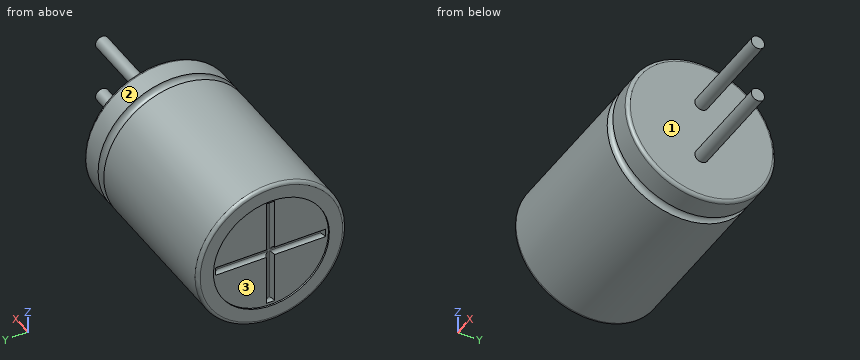
from build123d import *

# Parameters (mm, degrees)
SKETCH6_R           = 0.4
BOSS_EXTRUDE1_DEPTH = 6
CUT_EXTRUDE1_DEPTH  = 0.2
FILLET2_R           = 0.2


with BuildPart() as part:
    # Sketch1 → Revolve1 (revolve)
    with BuildSketch(Plane(origin=(0, 0, 0), x_dir=(1, 0, 0), z_dir=(0, 1, 0))):
        with BuildLine():
            Line((-5.95, -1.25), (-6.05, -1.25))
            Line((-6.05, -1.25), (-6.05, -2.25))
            Line((-6.05, -2.25), (-5.95, -2.25))
            Line((-5.95, -2.25), (3.85, -2.25))
            ThreePointArc((3.85, -2.25), (4.15, -1.95), (4.45, -2.25))
            Line((4.45, -2.25), (5.95, -2.25))
            Line((5.95, -2.25), (5.95, 2.25))
            Line((5.95, 2.25), (-5.95, 2.25))
            Line((-5.95, 2.25), (-5.95, -1.25))
        make_face()
    revolve(axis=Axis((-5.95, 0, -2.25), (1, 0, 0)))

    # Sketch6 → Boss-Extrude1 (add)
    with BuildSketch(Plane(origin=(5.95, 0, 0), x_dir=(0, 0, -1), z_dir=(1, 0, 0))):
        with Locations((0.5, 0)):
            Circle(SKETCH6_R)
        with Locations((4, 0)):
            Circle(SKETCH6_R)
    extrude(amount=BOSS_EXTRUDE1_DEPTH)

    # Sketch8 → Cut-Extrude1 (cut)
    with BuildSketch(Plane.ZY.offset(5.95)):
        Polygon((-2, -0.25), (-2, -3.325), (-2.5, -3.325), (-2.5, -0.25), (-5.575, -0.25), (-5.575, 0.25), (-2.5, 0.25), (-2.5, 3.325), (-2, 3.325), (-2, 0.25), (1.075, 0.25), (1.075, -0.25), align=None)
    extrude(amount=-CUT_EXTRUDE1_DEPTH, mode=Mode.SUBTRACT)

    # Fillet2
    fillet2_edges = [part.edges().sort_by_distance(p)[0] for p in [
        (-5.75, -3.325, -2.25),
        (-5.75, -1.7875, -2.5),
        (-5.75, -0.25, -4.0375),
        (-5.75, 0, -5.575),
        (-5.75, 0.25, -4.0375),
        (-5.75, 1.7875, -2.5),
        (-5.75, 3.325, -2.25),
        (-5.75, 1.7875, -2),
        (-5.75, 0.25, -0.4625),
        (-5.75, 0, 1.075),
        (-5.75, -0.25, -0.4625),
        (-5.75, -1.7875, -2),
        (5.95, 0, -6.75),
        (-6.05, 0, -6.75),
    ]]
    fillet(fillet2_edges, radius=FILLET2_R - 0.0001)  # a hair under: the kernel refuses the full size


solid = part.part
Geometry check sheet. Reference: the model listing, model coordinates, mm. Face numbers are marked on the shaded views. Give positions to 0.01 mm unless a question says otherwise; leave off trailing zeros. Write each loop counter-clockwise with the first axis right and the second up, starting at its lowest first coordinate (ties: lowest second). Pieces come first, ordered by that corner, then holes. Notation, with made-up numbers: (63.25, 36.5) - (118.25, 36.5) arc R32 cw to (118.25, 73.5) - close; hole circle Ø2 at (16, -9). An arc over 180 degrees is marked (long way). Put each result on its own line as item: value.
1. Draft check along Y on the marked faces 1, 2 and 3. Enter one of: +Y half, -Y half, draft (parallel to the pull), parting line (faces both ways), or undercut.
Ans:
face 1: draft
face 2: parting line
face 3: undercut
2. Thickness scan on line 1 (X direction, y = 2.25, z = -4.75); line 2 (Z direction, x = -6, y = 0); line 3 (X direction, y = 3, z = -5.5). Record the ranges inside material, lowest first.
Ans:
line 1: x = -5.95 to 5.95
line 2: z = -6.68 to -5.75, 1.25 to 2.18
line 3: x = -6.01 to 3.86, 4.44 to 5.91
3. Sectioned sample at A-A, the plane x = 9. Enter the section's corners in (y, z), plus the area to 3 significant figures.
Ans:
outline: circle Ø0.8 at (0, -4); circle Ø0.8 at (0, -0.5)
area: 1.01 mm²
4. Sectioned sample at B-B, the plane x = -3.5. Enter the section's corners in (y, z), plus the area to 3 significant figures.
Ans:
outline: circle Ø9 at (0, -2.25)
area: 63.6 mm²
5. Go/stop test with flat-tipped pins: pin 1 (1.9 mm diameter, centred on y = -0.5, z = -3.5, fed in from -X); pin 2 (2 mm diameter, centred on x = 4.5, z = -5.5, fed in from -Y); pin 3 (1 mm diameter, centred on y = 2.5, z = -1, fed in from +X). Record where each tip stops, or that it passes through.
Ans:
pin 1: stops at x = -5.95
pin 2: stops at y = -3.9
pin 3: stops at x = 5.95
